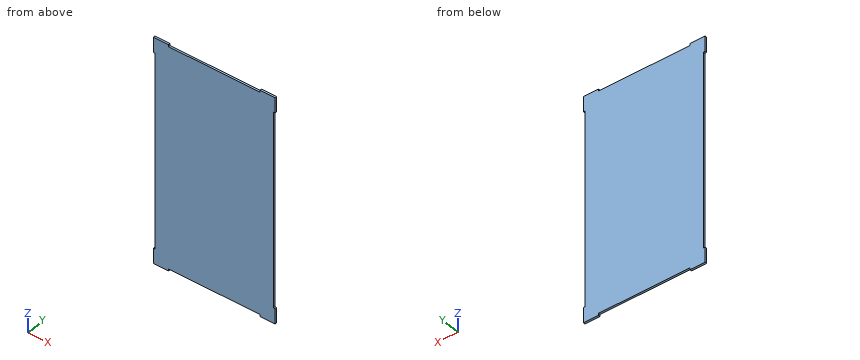
Autodesk Inventor part; units mm, degrees
ref_plane "YZ Plane" through (0, 0, 0) normal (1, 0, 0) x (0, 1, 0)
ref_plane "XZ Plane" through (0, 0, 0) normal (0, 1, 0) x (-1, 0, 0)
ref_plane "XY Plane" through (0, 0, 0) normal (0, 0, 1) x (1, 0, 0)
sketch "Sketch1" plane through (0, 0, 0) normal (0, 1, 0) x (-1, 0, 0)
  line L0 (-101.6, 190.5) -> (101.6, 190.5)
  line L1 (101.6, 190.5) -> (101.6, -190.5)
  line L2 (101.6, -190.5) -> (-101.6, -190.5)
  line L3 (-101.6, -190.5) -> (-101.6, 190.5)
  line L4 (-101.6, 190.5) -> (101.6, -190.5) construction
  line L5 (101.6, 190.5) -> (-101.6, -190.5) construction
  point P0 (0, 0)
  dimension "d0" = 203.2
  dimension "d1" = 381
extrude "Extrusion1" add sketch "Sketch1" along normal blind 3.175
sketch "Sketch2" plane through (0, 3.175, 0) normal (0, 1, 0) x (1, 0, 0)
  line L0 (-76.2, -190.5) -> (-76.2, -187.325)
  line L1 (-101.6, -165.1) -> (-98.425, -165.1)
  line L2 (-98.425, -165.1) -> (-98.425, 0)
  line L3 (-76.2, -187.325) -> (0, -187.325)
  line L4 (-101.6, 190.5) -> (-101.6, 165.1)
  line L5 (-101.6, 165.1) -> (-98.425, 165.1)
  line L6 (-98.425, 165.1) -> (-98.425, 0)
  line L7 (-101.6, 190.5) -> (-76.2, 190.5)
  line L8 (0, -187.325) -> (76.2, -187.325)
  line L9 (76.2, -187.325) -> (76.2, -190.5)
  line L10 (101.6, -190.5) -> (101.6, -165.1)
  line L11 (101.6, -190.5) -> (101.6, 190.5)
  line L12 (101.6, -165.1) -> (98.425, -165.1)
  line L13 (98.425, -165.1) -> (98.425, 165.1)
  line L14 (98.425, 165.1) -> (101.6, 165.1)
  line L15 (-76.2, 190.5) -> (-76.2, 187.325)
  line L16 (-76.2, 187.325) -> (76.2, 187.325)
  line L17 (76.2, 187.325) -> (76.2, 190.5)
  line L18 (76.2, 190.5) -> (-76.2, 190.5)
  line L19 (101.6, -165.1) -> (142.875, -125.4125)
  line L20 (142.875, -125.4125) -> (138.1125, 114.3)
  line L21 (138.1125, 114.3) -> (101.6, 165.1)
  line L22 (-76.2, -190.5) -> (66.675, -207.9625)
  line L23 (66.675, -207.9625) -> (76.2, -190.5)
  line L24 (-101.6, -165.1) -> (-173.0375, -100.0125)
  line L25 (-173.0375, -100.0125) -> (-152.4, 165.1)
  line L26 (-152.4, 165.1) -> (-101.6, 165.1)
  point P0 (-101.6, -190.5)
  dimension "d5" = 25.4
  dimension "d6" = 76.2
  dimension "d7" = 180
extrude "Extrusion2" cut sketch "Sketch2" against normal blind 3.175 contours L0 L3 L8 L9 L23 L22 | L24 L25 L26 L5 L6 L2 L1 | L18 L17 L16 L15 | L12 L13 L14 L11
properties part number "bottom"
The listing builds one solid part. Answer for the finished solid, in the listing's coordinates (mm). Give positions to 0.01 mm unless a question says otherwise; leave off trailing zeros. Loops run counter-clockwise (first coordinate to the right, second up) from the corner with the lowest first, then second, coordinate; pieces in that order, holes last. Notation, with made-up numbers: M 76.5,77.25 L 84.5,77.25 A31 cw 84.5,108.25 Z; hole C 80.25,11 d7. An arc over 180 degrees is marked long. Answer as CSV lines item,"result".
Item 1: The part is cut by section A-A (y = 1.3). Give the vertices of the cut face in (x, z) (3 decimals).
Values follow:
outline,"M -101.6,-190.5 L -76.2,-190.5 L -76.2,-187.325 L 76.2,-187.325 L 76.2,-190.5 L 101.6,-190.5 L 101.6,-165.1 L 98.425,-165.1 L 98.425,165.1 L 101.6,165.1 L 101.6,190.5 L 76.2,190.5 L 76.2,187.325 L -76.2,187.325 L -76.2,190.5 L -101.6,190.5 L -101.6,165.1 L -98.425,165.1 L -98.425,-165.1 L -101.6,-165.1 Z"
Item 2: Given pin 1 Ø1.6 at (x, y) = (22.5, 2) entering from +Z (3 decimals); pin 2 Ø1.5 at (x, y) = (68.5, 2.5) entering from -Z (3 decimals); pin 3 Ø1.6 at (y, z) = (1.5, 49.5) entering from -X (3 decimals), each flat-ended and moving along its own axis, determine where each tip first touches the part or whether it passes through.
Values follow:
pin 1,"stops at z = 187.325"
pin 2,"stops at z = -187.325"
pin 3,"stops at x = -98.425"
Item 3: The part is cut by section C-C (z = 82). Give the vertices of the cut face in (x, y) (3 decimals), and give its area (3 significant figures).
Values follow:
outline,"M -98.425,0 L 98.425,0 L 98.425,3.175 L -98.425,3.175 Z"
area,"625 mm^2"
Item 4: Straight lines are drawn through the part: line 1 along X through (y, z) = (2.75, 47.5) (3 decimals); line 2 along Z through (x, y) = (5.5, 0.9) (3 decimals). For each, find the intervals that lie inside material, in ascending order. Write a range as [from, to].
Values follow:
line 1,"x = [-98.425, 98.425]"
line 2,"z = [-187.325, 187.325]"
Item 5: The part is cut by section B-B (x = 17.5). Give the vertices of the cut face in (y, z) (3 decimals), and give its area (3 significant figures).
Values follow:
outline,"M 0,-187.325 L 3.175,-187.325 L 3.175,187.325 L 0,187.325 Z"
area,"1,190 mm^2"
